from build123d import *

# Parameters (mm, degrees)
SKETCH1_R           = 50
BOSS_EXTRUDE1_DEPTH = 200
BOSS_EXTRUDE2_DEPTH = 100
BOSS_EXTRUDE4_DEPTH = 86.60254
CIRPATTERN1_COUNT   = 3


with BuildPart() as part:
    # Sketch1 → Boss-Extrude1 (new body)
    with BuildSketch(Plane.XY):
        Circle(SKETCH1_R)
    extrude(amount=BOSS_EXTRUDE1_DEPTH)

    # Sketch2 → Boss-Extrude2 (add)
    with BuildSketch(Plane.XY.offset(200)):
        Polygon((43.301270189, 25), (43.301270189, 75), (-43.301270189, 75), (-43.301270189, 25), (0, 0), align=None)
    boss_extrude2 = extrude(amount=BOSS_EXTRUDE2_DEPTH)

    # Sketch3 → Boss-Extrude4 (add)
    with BuildSketch(Plane(origin=(-43.301270189, 0, 0), x_dir=(0, 1, 0), z_dir=(-1, 0, 0))):
        Polygon((75, -200), (75, -500), (125, -400), (125, -300), align=None)
    boss_extrude4 = extrude(amount=-BOSS_EXTRUDE4_DEPTH)

    # CirPattern1: Boss-Extrude2, Boss-Extrude4 ×3 about axis
    cirpattern1_axis = Axis((0, 0, 0), (0, 0, 1))
    for i in range(1, CIRPATTERN1_COUNT):
        add(boss_extrude2.rotate(cirpattern1_axis, i * 360 / CIRPATTERN1_COUNT))
        add(boss_extrude4.rotate(cirpattern1_axis, i * 360 / CIRPATTERN1_COUNT))


solid = part.part
CAD build for the part. Positions are in the model's coordinates, mm. A direction names the side the tool comes from. Give positions to 0.01 mm unless a question says otherwise; leave off trailing zeros. Loops run counter-clockwise (first coordinate to the right, second up) from the corner with the lowest first, then second, coordinate; pieces in that order, holes last. Notation, with made-up numbers: M 83,14.25 L 102,14.25 A31 ccw 102,45.25 Z; hole C 25,13 d6. An arc over 180 degrees is marked long. One line per question, with ' | ' between items. Start each with the question number.
1. Probe L1, parallel to Z at x = 31.5, y = -16; L2, parallel to X at y = -68, z = 286; L3, parallel to X at y = -71, z = 268.5. List the from-to ranges inside material, lowest first. Write a range as from..to.
2. Two-plate mould, pull along X, no slides. Class faces 5 (the face through (86.6, -49.3, 450.7)), 6 (the face through (-52.318, -80.206, 314.567)), 7 (the face through (47.69, 15.02, 98.6)), 8 (the face through (-1, 125, 351)): pulls with the +X half, pulls with the -X half, needs draft (parallel to the pull), parting line crosses it, or undercut.
3. 3-axis set-ups, long thin cutter, end or side, ignore diameter. For faces 1 (the face through (2, 1, 300)), 2 (the face through (-0.61, 99.65, 450.7)), 3 (the face through (-1, 75, 399)), 4 (the face through (-43.301, 85, 315)): which of +Z, -Z, +X, -X, +Y, -Y reach the whole face in a straight line?
4. Flat gauge pins, fed straight in: pin 1 (3 mm diameter, centred on x = 75.5, y = -73.5, fed in from +Z); pin 2 (12 mm diameter, centred on x = -60, y = -46.5, fed in from +Z); pin 3 (1.5 mm diameter, centred on x = -18.5, z = 104, fed in from +Y). Where does each tip first touch, or does it go through?
5. Saw through at B-B on y = -14. Give the cut face in (x, z).
6. Saw through at C-C on x = -96. Give the cut face in (y, z), plus the area to 3 significant figures.
7. Saw through at D-D on y = 102. Give the cut face in (x, z).
8. Saw through at A-A on y = -57.5. Give the cut face in (x, z).
Result sheet:
1) L1: z = 0..300 | L2: x = -96.99..-31.18, 31.18..96.99 | L3: x = -85.16..-36.37, 36.37..85.16
2) face 5: pulls with the +X half | face 6: undercut | face 7: parting line crosses it | face 8: needs draft
3) face 1: +Z | face 2: +Z, +X, -X, +Y | face 3: +Z, +X, -X, -Y | face 4: +Z, -Z, -X, +Y
4) pin 1: stops at z = 448.73 | pin 2: stops at z = 500 | pin 3: stops at y = 46.74
5) outline: M -110.85,256 L -78.52,200 L -48,200 L -48,0 L 48,0 L 48,200 L 78.52,200 L 110.85,256 L 110.85,444 L 78.52,500 L 78.52,300 L -78.52,300 L -78.52,500 L -110.85,444 Z
6) outline: M -83.72,300 L -5.43,221.7 L -5.43,478.3 L -83.72,400 Z | area: 14,000 mm^2
7) outline: M -43.3,254 L 43.3,254 L 43.3,446 L -43.3,446 Z
8) outline: M -111.14,300 L -53.4,200 L -12.99,200 L -12.99,300 L -53.4,300 L -53.4,500 L -111.14,400 Z; M 12.99,200 L 53.4,200 L 111.14,300 L 111.14,400 L 53.4,500 L 53.4,300 L 12.99,300 Z
